Geometry: final body of the model. Coordinates: model frame, mm. A direction names the side the tool comes from. Give positions to 0.01 mm unless a question says otherwise; leave off trailing zeros. Write each loop counter-clockwise with the first axis right and the second up, starting at its lowest first coordinate (ties: lowest second). Pieces come first, ordered by that corner, then holes. Notation, with made-up numbers: M -13.75,89 L 27.25,89 A28 cw 27.25,108 Z; hole C 32,32 d9. An arc over 180 degrees is marked long. Use a Markdown table: item, result. Add a question column.
1) Section A-A on y = 0. Return the cut outline in (x, z).
2) Line query: line 1 (Y direction, x = 0, z = 0.75); line 2 (Z direction, x = -3.5, y = 2.25); line 3 (X direction, y = -6.25, z = -0.4). Output: solid intervals per line, ascending.
3) Pin query (flat end, axial travel): pin 1 (1.5 mm diameter, centred on x = 2, z = 0.5, fed in from +Y); pin 2 (1 mm diameter, centred on y = -4.5, z = -0.5, fed in from -X); pin 3 (1.5 mm diameter, centred on x = -0.5, y = 0, fed in from +Z). Return the tip coordinate at first contact, or that it passes through.
4) Set-up query: faces 1 (the flat face through (2, 0, 2)), 2 (the cylindrical face through (-1.5, 0.07, 1.01)). Return all of +Z, -Z, +X, -X, +Y, -Y with unobstructed straight access to the full face (end or side cutting, diameter ignored); none if empty.
5) Draft query along X for faces 3 (the flat face through (0, 0, 0)), 4 (the flat face through (-3, -3, 0)), 5 (the cylindrical face through (7.493, 0.33, -0.493)). Return one class per face: +X half, -X half, draft (parallel to the pull), parting line (faces both ways), or undercut.
6) Section C-C on z = 1.4. Return the cut outline in (x, y).
7) Section D-D on z = -0.65. Return the cut outline in (x, y).
```python
from build123d import *

# Parameters (mm, degrees)
ESQUISSE1_R             = 4
BOSS_EXTRU_1_DEPTH      = 2
ESQUISSE2_R             = 1.5
ENL_V_MAT_EXTRU_1_DEPTH = 2.5
ESQUISSE3_R             = 7.5
BOSS_EXTRU_2_DEPTH      = 1


with BuildPart() as part:
    # Esquisse1 → Boss.-Extru.1 (new body)
    with BuildSketch(Plane.XY):
        Circle(ESQUISSE1_R)
    extrude(amount=BOSS_EXTRU_1_DEPTH)

    # Esquisse2 → Enlèv. mat.-Extru.1 (cut)
    with BuildSketch(Plane.XY.offset(2)):
        Circle(ESQUISSE2_R)
    extrude(amount=-ENL_V_MAT_EXTRU_1_DEPTH, mode=Mode.SUBTRACT)

    # Esquisse3 → Boss.-Extru.2 (add)
    with BuildSketch(Plane(origin=(0, 0, 0), x_dir=(-1, 0, 0), z_dir=(0, 0, -1))):
        Circle(ESQUISSE3_R)
    extrude(amount=BOSS_EXTRU_2_DEPTH)


solid = part.part
```
Found:
| question | item | result |
|---|---|---|
| 1 | outline | M -7.5,-1 L 7.5,-1 L 7.5,0 L 4,0 L 4,2 L 1.5,2 L 1.5,0 L -1.5,0 L -1.5,2 L -4,2 L -4,0 L -7.5,0 Z |
| 2 | line 1 | -4 to -1.5, 1.5 to 4 |
| 2 | line 2 | -1 to 0 |
| 2 | line 3 | -4.15 to 4.15 |
| 3 | pin 1 | y = 7.36 |
| 3 | pin 2 | x = -6.34 |
| 3 | pin 3 | z = 0 |
| 4 | face 1 | +Z, +X, -X, +Y, -Y |
| 4 | face 2 | +Z |
| 5 | face 3 | undercut |
| 5 | face 4 | draft |
| 5 | face 5 | parting line |
| 6 | outline | C 0,0 d8; hole C 0,0 d3 |
| 7 | outline | C 0,0 d15 |
